The listing builds one solid part. Answer for the finished solid, in the listing's coordinates (mm). Face numbers are marked on the shaded views. Give positions to 0.01 mm unless a question says otherwise; leave off trailing zeros. Write each loop counter-clockwise with the first axis right and the second up, starting at its lowest first coordinate (ties: lowest second). Pieces come first, ordered by that corner, then holes.
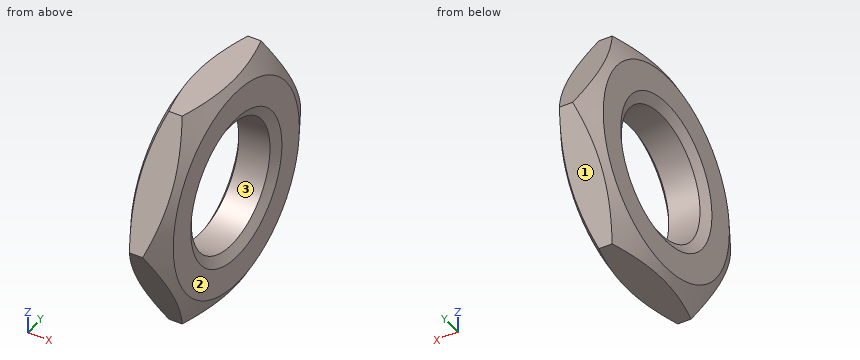
Autodesk Inventor part; units mm, degrees
ref_plane "Work Plane1" through (-48.5942, 0, 0) normal (0, -0.866, -0.5) x (1, 0, 0)
ref_plane "YZ Plane" through (0, 0, 0) normal (1, 0, 0) x (0, 1, 0)
ref_plane "XZ Plane" through (0, 0, 0) normal (0, 1, 0) x (-1, 0, 0)
sketch "Sketch1" plane through (0, 0, 0) normal (1, 0, 0) x (0, 1, 0)
  line L0 (-20.7846, 0) -> (-10.3923, 18)
  line L1 (-10.3923, 18) -> (10.3923, 18)
  line L2 (10.3923, 18) -> (20.7846, 0)
  line L3 (20.7846, 0) -> (10.3923, -18)
  line L4 (10.3923, -18) -> (-10.3923, -18)
  line L5 (-10.3923, -18) -> (-20.7846, 0)
  point P0 (0, 0)
  point P1 (0, 0)
  dimension "d0" = 41.5692
extrude "Body" add sketch "Sketch1" along normal blind 7
sketch "Sketch2" plane through (0, 0, 0) normal (0, 0, 1) x (1, 0, 0)
  line L0 (0, 10.3923) -> (0, 20.7846)
  line L1 (0, 20.7846) -> (7, 20.7846)
  line L2 (7, 10.3923) -> (7, 20.7846)
  line L3 (-2.4, 0) -> (14.4, 0)
  line L4 (2.416, 20.7846) -> (0, 16.6)
  line L5 (4.584, 20.7846) -> (7, 16.6)
  dimension "d3" = 30
  dimension "d4" = 30
  dimension "d5" = 33.2
  dimension "d6" = 33.2
revolve "Chamfer1" cut sketch "Sketch2" angle 360 about axis through (-10, 0, 0) along (1, 0, 0)
sketch "Sketch3" plane through (7, 0, 0) normal (1, 0, 0) x (0, 0, -1)
  arc A0 (-0.625, -1.0825) -> (0.625, -1.0825) centre (0, 0) ccw
hole "Thread" at (7, 0, 0) direction (-1, 0, 0) diameter 20.752 end through all
chamfer "Chamfer2" distance 1.6238 angle 30 1 edges at (7, 0, 10.376) measured on face at (7, 14.3393, -1.7411)
chamfer "Chamfer3" distance 1.6238 angle 30 1 edges at (0, 0, 10.376) measured on face at (0, 14.3393, -1.7411)
ref_plane "Work Plane1" through (-48.5942, 0, 0) normal (0, -0.866, -0.5) x (1, 0, 0)
equation "\"d0\" = 1.1547 * SW"
equation "\"d3\" = ANG1"
equation "\"d4\" = ANG2"
equation "\"d5\" = SW0"
equation "\"d6\" = SW01"
equation "\"d8\" = -0.5 * GD1 + 0.5 * NND"
equation "\"d40\" = -0.5 * GD1 + 0.5 * NND"
equation "\"d10\" = -0.5 * GD1 + 0.5 * NND"
equation "\"d41\" = -0.5 * GD1 + 0.5 * NND"
equation "\"ANG1\" = 30deg"
equation "\"ANG2\" = 30deg"
equation "\"NND\" = 24"
equation "\"KOH\" = 12"
equation "\"SW\" = 36"
equation "\"SW0\" = 33.2"
equation "\"SW01\" = SW0"
equation "\"GUL\" = 0.541266 * PTC"
equation "\"THREADDIA\" = 24"
equation "\"TOA\" = 30deg"
equation "\"PTC\" = 3"
equation "\"E0\" = 1.155 * SW"
equation "\"GAL\" = 0.541266 * PTC"
properties part number "PWTR-0062" material "Stainless Steel, 440C"
Item 1: Consider probe 1 along Y at (x, z) = (3.85, 0); probe 2 along Y at (x, z) = (2.2, 0); probe 3 along Z at (x, y) = (3.65, 0). Determine where each line is inside the solid, lowest interval first.
Conclusion:
probe 1: y = -20.78 to -10.38, 10.38 to 20.78
probe 2: y = -20.41 to -10.38, 10.38 to 20.41
probe 3: z = -18 to -10.38, 10.38 to 18
Item 2: Each of these flat-tipped pins is pushed along its axis until it touches: P1, Ø5, axis at y = 8.5, z = 4, coming from the -X side; P2, Ø1, axis at x = 1.5, y = -10, coming from the -Z side. Where does it stop, or does it pass through?
Conclusion:
P1: stops at x = 0.06
P2: stops at z = -17.43
Item 3: A cutting plane is placed at A-A, the plane y = 0. Give the vertices of the cut face in (x, z), plus the area to 3 significant figures.
Conclusion:
outline: (0, -16.6) - (0.81, -18) - (6.19, -18) - (7, -16.6) - (7, -12) - (6.06, -10.38) - (0.94, -10.38) - (0, -12) - close; (0, 12) - (0.94, 10.38) - (6.06, 10.38) - (7, 12) - (7, 16.6) - (6.19, 18) - (0.81, 18) - (0, 16.6) - close
area: 101 mm2
Item 4: A cutting plane is placed at B-B, the plane x = 3.75. Give the vertices of the cut face in (y, z), plus the area to 3 significant figures.
Conclusion:
outline: (-20.78, 0) - (-10.39, -18) - (10.39, -18) - (20.78, 0) - (10.39, 18) - (-10.39, 18) - close; hole circle Ø20.75 at (0, 0)
area: 784 mm2
Item 5: Determine the mould class of the marked faces 1, 2 and 3 for opening direction Y: pulls with the +Y half, pulls with the -Y half, needs draft (parallel to the pull), parting line crosses it, or undercut.
Conclusion:
face 1: pulls with the +Y half
face 2: needs draft
face 3: undercut
